Check sheet for the modelled part. Datum: model origin and axes. Units: mm. A direction names the side the tool comes from. Round coordinates to 2 decimals unless told otherwise and drop trailing zeros. Write each loop counter-clockwise with the first axis right and the second up, starting at its lowest first coordinate (ties: lowest second). Pieces come first, ordered by that corner, then holes.
Item 1: Release check for a two-part mould opening along Z. For faces 1 (the flat face through (1.109, -0.139, 8.042)), 2 (the flat face through (2.25, 0, 10)), 3 (the flat face through (0, 0, 0)), 4 (the flat face through (0, 0, 20)) record: pulls with the +Z half, pulls with the -Z half, needs draft (parallel to the pull), parting line crosses it, or undercut.
Item 2: Section check D-D, the plane y = 3. Record the cut outline in (x, z), plus the area to 3 significant figures.
Item 3: Depth check by flat-ended pin: pin 1 (2 mm diameter, centred on y = -4.5, z = 10, fed in from -X); pin 2 (3 mm diameter, centred on y = 4, z = 10.5, fed in from +X). Enter the tip coordinate at first touch or a pass-through.
Item 4: Set-up check for faces 5 (the flat face through (-1.14, -0.14, 8.06)), 6 (the cylindrical face through (9.443, 2.974, 9.86)): record each of +Z, -Z, +X, -X, +Y, -Y from which the full face is reachable in a straight line by a thin tool's end or side.
Item 5: Section check B-B, the plane x = 1. Record the cut outline in (y, z), plus the area to 3 significant figures.
Item 6: Section check C-C, the plane z = 1.5. Record the cut outline in (x, y), plus the area to 3 significant figures.
Item 7: Section check A-A, the plane y = 0. Record the cut outline in (x, z), plus the area to 3 significant figures.
Item 8: Material ranges on line 1 along X through (y, z) = (-4.5, 10.5); line 2 along X through (y, z) = (3.75, 7.5); line 3 along Z through (x, y) = (1.5, 4.5), recorded low to high.
from build123d import *

# Parameters (mm, degrees)
F0_R          = 9.9
F1_DEPTH      = 20
F3_DEPTH      = 9.901
F3_DEPTH_BACK = 9.901


with BuildPart() as f1:
    # F0 (on Top) → F1 (new body)
    with BuildSketch(Plane.XY):
        Circle(F0_R)
    extrude(amount=F1_DEPTH)

    # F2 (on Front) → F3 (cut, two sides)
    with BuildSketch(Plane.XZ) as f3_sk:
        Polygon((2.25, 8.7009618943), (2.25, 11.2990381057), (0, 12.5980762114), (-2.25, 11.2990381057), (-2.25, 8.7009618943), (0, 7.4019237886), align=None)
    extrude(amount=-F3_DEPTH, mode=Mode.SUBTRACT)
    extrude(f3_sk.sketch, amount=F3_DEPTH_BACK, mode=Mode.SUBTRACT)


solid = f1.part
Values found:
1. face 1: undercut
1. face 2: undercut
1. face 3: pulls with the -Z half
1. face 4: pulls with the +Z half
2. outline: (-9.43, 0) - (9.43, 0) - (9.43, 20) - (-9.43, 20) - close; hole (-2.25, 8.7) - (0, 7.4) - (2.25, 8.7) - (2.25, 11.3) - (0, 12.6) - (-2.25, 11.3) - close
2. area: 360 mm2
3. pin 1: stops at x = -9.26
3. pin 2: stops at x = 9.58
4. face 5: +Y, -Y
4. face 6: +Z, -Z
5. outline: (-9.85, 0) - (9.85, 0) - (9.85, 7.98) - (-9.85, 7.98) - close; (-9.85, 12.02) - (9.85, 12.02) - (9.85, 20) - (-9.85, 20) - close
5. area: 314 mm2
6. outline: circle Ø19.8 at (0, 0)
6. area: 308 mm2
7. outline: (-9.9, 0) - (9.9, 0) - (9.9, 20) - (-9.9, 20) - close; hole (-2.25, 8.7) - (0, 7.4) - (2.25, 8.7) - (2.25, 11.3) - (0, 12.6) - (-2.25, 11.3) - close
7. area: 378 mm2
8. line 1: x = -8.82 to -2.25, 2.25 to 8.82
8. line 2: x = -9.16 to -0.17, 0.17 to 9.16
8. line 3: z = 0 to 8.27, 11.73 to 20
